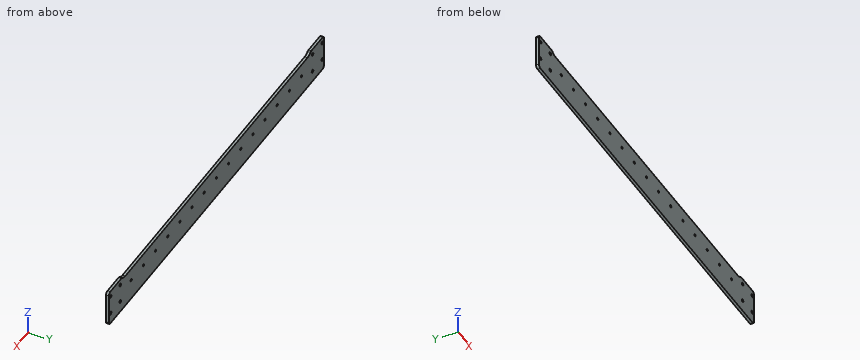
```python
from build123d import *

# Parameters (mm, degrees)
BOSS_EXTRUDE1_DEPTH                   = 3
M3_CLEARANCE_HOLE1_D                  = 3.2
M3_CLEARANCE_HOLE1_CSINK_D            = 3.25
M3_CLEARANCE_HOLE1_CSINK_ANGLE        = 90
FILLET1_R                             = 10
FILLET2_R                             = 3
TAP_DRILL_FOR_M3X0_5_TAP2_D           = 2.5
TAP_DRILL_FOR_M3X0_5_TAP2_CSINK_D     = 2.55
TAP_DRILL_FOR_M3X0_5_TAP2_CSINK_ANGLE = 90
LPATTERN1_COUNT                       = 15
LPATTERN1_PITCH                       = 25


with BuildPart() as part:
    # Sketch1 → Boss-Extrude1 (new body)
    with BuildSketch(Plane(origin=(0, 0, 0), x_dir=(1, 0, 0), z_dir=(0, 1, 0))):
        Polygon((0, 0), (194, 0), (194, -2.7), (221, -2.7), (221, 29.7), (221, 35.5), (0, 35.5), (0, 29.7), align=None)
    extrude(amount=BOSS_EXTRUDE1_DEPTH)

    # M3 Clearance Hole1 (through all)
    with Locations(Plane(origin=(0, 3, 0), x_dir=(1, 0, 0), z_dir=(0, 1, 0))):
        with Locations((197.5, 23.5), (217.5, 3.5), (217.5, 23.5), (197.5, 3.5)):
            CounterSinkHole(M3_CLEARANCE_HOLE1_D / 2, M3_CLEARANCE_HOLE1_CSINK_D / 2, counter_sink_angle=M3_CLEARANCE_HOLE1_CSINK_ANGLE)

    # Fillet1
    # the kernel refuses this fillet: 10 mm, written as the material it adds along each edge
    with BuildSketch(Plane(origin=(194, 0, 0), x_dir=(-1, 0, 0), z_dir=(0, 1, 0))) as fillet1_piece_1:
        with BuildLine():
            CenterArc((6.83447145, 10), FILLET1_R, 226.886394054, 43.113605946)
            Line((0, 2.7), (-0.136689429, 2.554))
            ThreePointArc((-0.136689429, 2.554), (-0.2, 1.35), (-0.2, 0))
            Line((-0.2, 0), (0, -0.2))
            Line((0, -0.2), (6.83447145, -0.2))
            Line((6.83447145, -0.2), (6.83447145, 0))
        make_face()
    extrude(amount=3)

    # Fillet2
    fillet2_edges = [part.edges().sort_by_distance(p)[0] for p in [
        (221, 1.5, -35.5),
        (221, 1.5, 2.7),
        (194, 1.5, 2.7),
    ]]
    fillet(fillet2_edges, radius=FILLET2_R)

    # Mirror1: part across plane


with BuildPart() as part_1:
    add(part.part)
    add(part.part.mirror(Plane(origin=(0, 3, -35.5), x_dir=(0, 0, 1), z_dir=(1, 0, 0))))

    # Tap Drill for M3x0.5 Tap2 (through all)
    with Locations(Plane(origin=(0, 0, 0), x_dir=(-1, 0, 0), z_dir=(0, -1, 0))):
        with Locations((-175, 13.5)):
            tap_drill_for_m3x0_5_tap2 = CounterSinkHole(TAP_DRILL_FOR_M3X0_5_TAP2_D / 2, TAP_DRILL_FOR_M3X0_5_TAP2_CSINK_D / 2, counter_sink_angle=TAP_DRILL_FOR_M3X0_5_TAP2_CSINK_ANGLE)

    # LPattern1: Tap Drill for M3x0.5 Tap2 ×15
    with Locations(*[(-i * LPATTERN1_PITCH, 0, 0) for i in range(1, LPATTERN1_COUNT)]):
        add(tap_drill_for_m3x0_5_tap2, mode=Mode.SUBTRACT)


solid = part_1.part
```
The model under review builds one solid part; all positions refer to its coordinate system, in mm. Round coordinates to 2 decimals unless told otherwise and drop trailing zeros. Order: outer loops, then holes, each group sorted by start corner. A loop starts at its lowest first (then second) coordinate and runs counter-clockwise, first axis right, second up.
(1) Wall thickness on L1, parallel to X at y = 0.65, z = -3; L2, parallel to Z at x = 197.5, y = 2.1; L3, parallel to Z at x = 25, y = 1.4: over which ranges is each line inside the solid? List them lowest first.
Working result:
L1: x = -221 to -219.02, -215.98 to -199.02, -195.98 to 195.98, 199.02 to 215.98, 219.02 to 221
L2: z = -35.5 to -25.1, -21.9 to -5.1, -1.9 to 2.7
L3: z = -35.5 to -14.75, -12.25 to 0
(2) Take a section at A-A, the plane x = 59.5. State the section outline as (y, z) points, plus the area to 4 significant figures.
Working result:
outline: (0, -35.5) - (3, -35.5) - (3, 0) - (0, 0) - close
area: 106.5 mm2
(3) For P1, Ø3.5, axis at x = -217.5, z = -3.5, coming from the +Y side, flat-tipped, find the tip position at first contact; note if it passes through.
Working result:
P1: stops at y = 3
(4) Take a section at B-B, the plane y = 1.5. Count the separate pieces of the cut face and the enclosed holes in it, plus the area to 3 significant figures.
Working result:
separate pieces: 1
enclosed holes: 23
area: 15,700 mm2
